For this review, use the dimensioned drawing (mm, ordinates from the lowest corner) and the shaded views. A direction names the side the tool comes from. Give positions to 0.01 mm unless a question says otherwise; leave off trailing zeros. Order: outer loops, then holes, each group sorted by start corner. A loop starts at its lowest first (then second) coordinate and runs counter-clockwise, first axis right, second up. Notation, with made-up numbers: (-27, 5.25) -> (-23, 5.25) arc R30 ccw to (-23, 35.25) -> close; hole circle Ø5 at (4.25, -11). An arc over 180 degrees is marked (long way). Return JSON: item names as keys, results as strings.
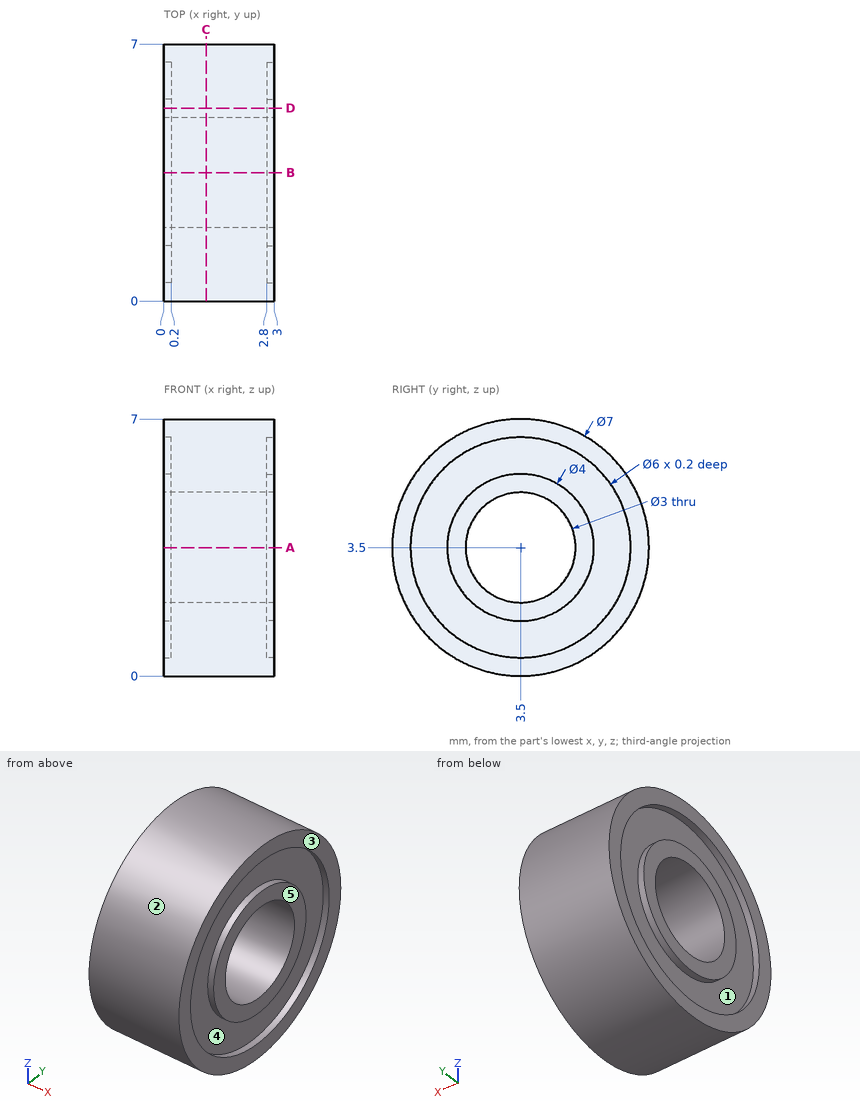
Item 1: Add section A-A (z = 3.5). Give the boundary of the cut face in (x, y).
Result set:
{"outline": "(0, 0) -> (3, 0) -> (3, 0.5) -> (2.8, 0.5) -> (2.8, 1.5) -> (3, 1.5) -> (3, 2) -> (0, 2) -> (0, 1.5) -> (0.2, 1.5) -> (0.2, 0.5) -> (0, 0.5) -> close; (0, 5) -> (3, 5) -> (3, 5.5) -> (2.8, 5.5) -> (2.8, 6.5) -> (3, 6.5) -> (3, 7) -> (0, 7) -> (0, 6.5) -> (0.2, 6.5) -> (0.2, 5.5) -> (0, 5.5) -> close"}
Item 2: Add section D-D (y = 5.25). Give the boundary of the cut face in (x, z).
Result set:
{"outline": "(0, 0.47) -> (3, 0.47) -> (3, 1.06) -> (2.8, 1.06) -> (2.8, 2.53) -> (3, 2.53) -> (3, 4.47) -> (2.8, 4.47) -> (2.8, 5.94) -> (3, 5.94) -> (3, 6.53) -> (0, 6.53) -> (0, 5.94) -> (0.2, 5.94) -> (0.2, 4.47) -> (0, 4.47) -> (0, 2.53) -> (0.2, 2.53) -> (0.2, 1.06) -> (0, 1.06) -> close"}
Item 3: Machinability: for the marked faces 4 and 5, which of the approach directions +Z, -Z, +X, -X, +Y, -Y give a long, thin tool a straight path to every point of the face, cutting with its end or side? Answer none if there is none.
Result set:
{"face 4": "+X", "face 5": "+Z, -Z, +X, +Y, -Y"}
Item 4: Wall thickness on L1, parallel to Z at x = 0.7, y = 3.5; L2, parallel to X at y = 4, z = 6.25; L3, parallel to Y at x = 0.1, z = 2.5: over which ranges is each line inside the solid? List them lowest first. Write a range as [from, to].
Result set:
{"L1": "z = [0, 2], [5, 7]", "L2": "x = [0.2, 2.8]", "L3": "y = [0.15, 0.67], [1.77, 2.38], [4.62, 5.23], [6.33, 6.85]"}
Item 5: For pin 1 (1.5 mm diameter, centred on x = 0.5, y = 5.5, fed in from -Z); pin 2 (1.5 mm diameter, centred on y = 2.5, z = 4.5, fed in from +X), all flat-tipped, find the tip position at first contact; note any pin that passes through.
Result set:
{"pin 1": "stops at z = 0.23", "pin 2": "stops at x = 3"}
Item 6: Add section C-C (x = 1.15). Give the boundary of the cut face in (y, z), plus the area to 3 significant figures.
Result set:
{"outline": "circle Ø7 at (3.5, 3.5); hole circle Ø3 at (3.5, 3.5)", "area": "31.4 mm^2"}
Item 7: Mouldability with a two-part tool opening along Z and no side actions: class the marked faces 1, 2 and 3 as released by +Z, released by -Z, zero draft, split by the parting line, or undercut.
Result set:
{"face 1": "undercut", "face 2": "split by the parting line", "face 3": "zero draft"}
